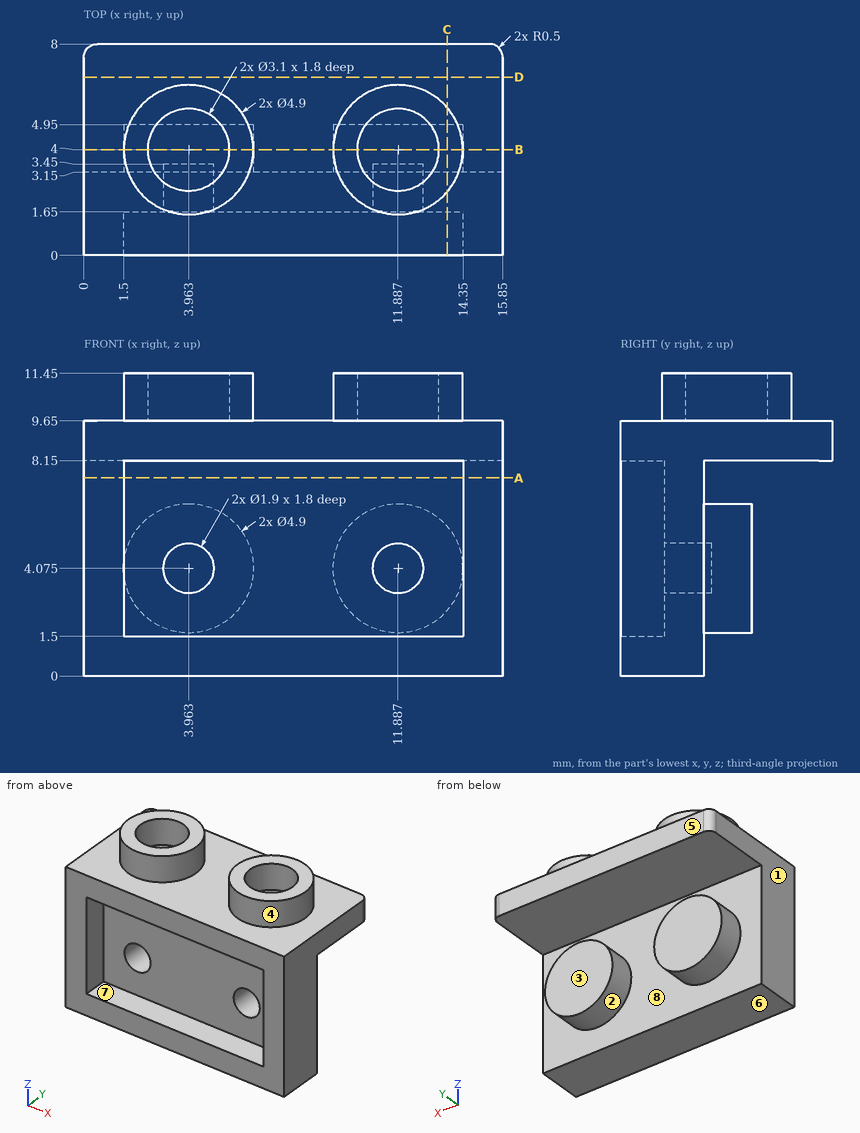
Part print with two shaded views. Sizes in mm from the minimum x, y, z corner. A direction names the side the tool comes from. Round coordinates to 2 decimals unless told otherwise and drop trailing zeros. Loops run counter-clockwise (first coordinate to the right, second up) from the corner with the lowest first, then second, coordinate; pieces in that order, holes last.
1. Drill centre lines: line 1 along Z through (x, y) = (5.25, 0.75); line 2 along Z through (x, y) = (9, 3.25); line 3 along Y through (x, z) = (11.25, 11) (1 decimal). Where is each one in solid material? Low to high.
Solutions:
line 1: z = 0 to 1.5, 8.15 to 9.65
line 2: z = 8.15 to 9.65
line 3: y = 1.6 to 2.6, 5.4 to 6.4
2. Slice it at A-A (z = 7.5). Give the cut face in (x, y).
Solutions:
outline: (0, 0) - (1.5, 0) - (1.5, 1.65) - (14.35, 1.65) - (14.35, 0) - (15.85, 0) - (15.85, 3.15) - (0, 3.15) - close
3. Flat gauge pins, fed straight in: pin 1 (1.5 mm diameter, centred on x = 3.5, z = 3.5, fed in from -Y); pin 2 (1.9 mm diameter, centred on x = 3.96, y = 4, fed in from +Z); pin 3 (1.5 mm diameter, centred on x = 3.5, z = 4, fed in from +Y). Where does each tip first touch, or does it go through?
Solutions:
pin 1: stops at y = 1.65
pin 2: stops at z = 9.65
pin 3: stops at y = 4.95
4. Slice it at B-B (y = 4). Count the separate pieces of the cut face and the enclosed holes in it.
Solutions:
separate pieces: 3
enclosed holes: 0
5. Slice it at D-D (y = 6.75). Give the cut face in (x, z).
Solutions:
outline: (0, 8.15) - (15.85, 8.15) - (15.85, 9.65) - (0, 9.65) - close
6. Slice it at C-C (x = 13.75). Give the cut face in (y, z).
Solutions:
outline: (0, 0) - (3.15, 0) - (3.15, 2.48) - (4.95, 2.48) - (4.95, 5.67) - (3.15, 5.67) - (3.15, 8.15) - (8, 8.15) - (8, 9.65) - (5.59, 9.65) - (5.59, 11.45) - (2.41, 11.45) - (2.41, 9.65) - (0, 9.65) - (0, 8.15) - (1.65, 8.15) - (1.65, 1.5) - (0, 1.5) - close
7. 3-axis set-ups, long thin cutter, end or side, ignore diameter. For the marked faces 4, 5, 6, 7 and 8: which of +Z, -Z, +X, -X, +Y, -Y reach the whole face in a straight line?
Solutions:
face 4: +Z
face 5: +Z, -Z, +X, -X, +Y
face 6: -Z, +X, -X, +Y, -Y
face 7: -Y
face 8: +Y
8. Two-plate mould, pull along X, no slides. Class the marked faces 1, 2 and 3: pulls with the +X half, pulls with the -X half, needs draft (parallel to the pull), parting line crosses it, or undercut.
Solutions:
face 1: pulls with the -X half
face 2: undercut
face 3: needs draft
